Study the drawing (mm; zero at the part's minimum x, y, z) and answer. Give positions to 0.01 mm unless a question says otherwise; leave off trailing zeros. Write each loop counter-clockwise with the first axis right and the second up, starting at its lowest first coordinate (ties: lowest second). Pieces come first, ordered by that corner, then holes. Notation, with made-up numbers: (-2, 49) -> (54, 49) arc R27 cw to (54, 76) -> close; hole circle Ø4 at (37.5, 30.25). An arc over 180 degrees is marked (long way). One line per question, with ' | ' between items.
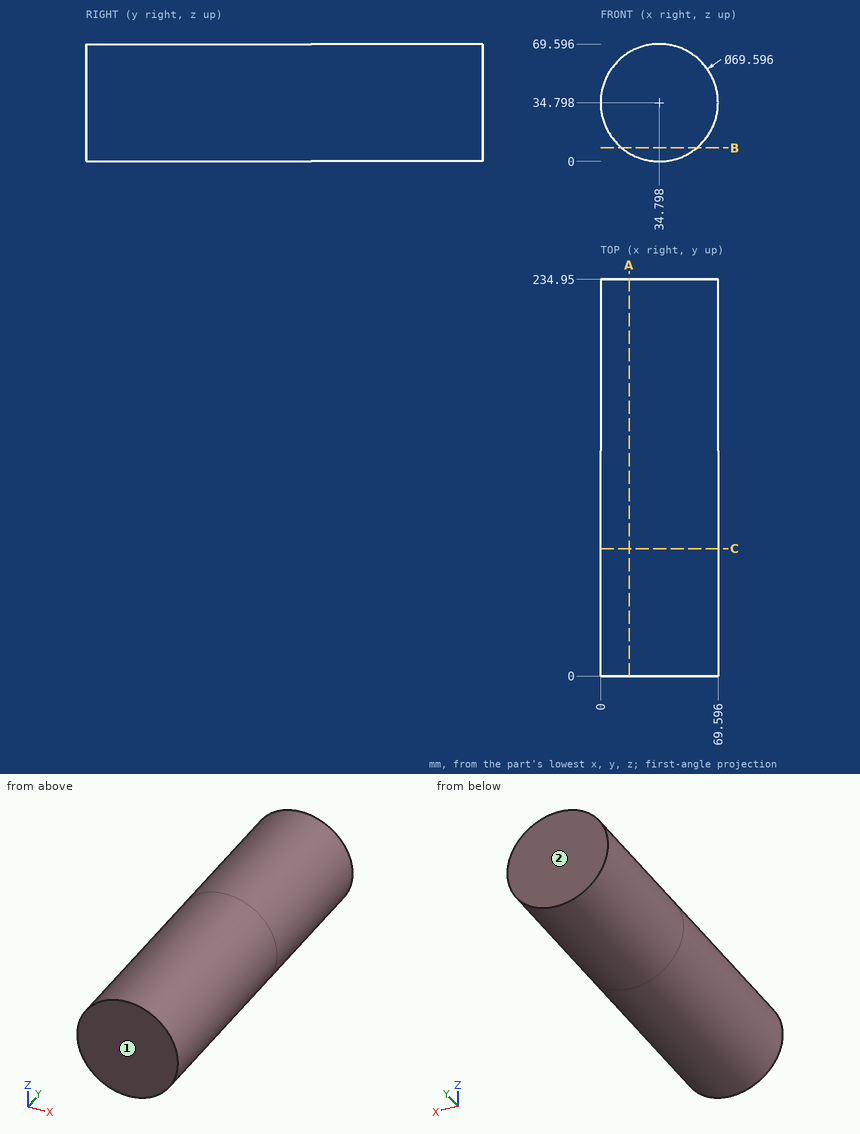
Item 1: Flat-ended cylindrical pins translate along their axes: pin 1 (1 mm diameter, centred on x = 17, y = 194.5, fed in from -Z); pin 2 (10 mm diameter, centred on x = 13, y = 118.5, fed in from +Z); pin 3 (6 mm diameter, centred on x = 24, y = 46, fed in from -Z) (3 decimals). Find the tip coordinate at first contact, or state that the pin passes through.
Answers below:
pin 1: z = 4.6 | pin 2: z = 65.27 | pin 3: z = 0.885
Item 2: Determine the mould class of the marked faces 1 and 2 for opening direction Y: pulls with the +Y half, pulls with the -Y half, needs draft (parallel to the pull), parting line crosses it, or undercut.
Answers below:
face 1: pulls with the -Y half | face 2: pulls with the +Y half
Item 3: Find section B-B (z = 8). Write down the section's boundary in (x, y).
Answers below:
outline: (12.6, 0) -> (57, 0) -> (57, 234.95) -> (12.6, 234.95) -> close
Item 4: Find section C-C (y = 75.5). Write down the section's boundary in (x, z), then the cut area to 3 significant figures.
Answers below:
outline: circle Ø69.6 at (34.8, 34.8) | area: 3,800 mm²
Item 5: Consider line 1 (Z direction, x = 35, y = 45); line 2 (X direction, y = 14, z = 34); line 3 (Z direction, x = 61, y = 206). Determine where each line is inside the solid, lowest interval first. Write a range as [from, to].
Answers below:
line 1: [0, 69.6] | line 2: [0.01, 69.59] | line 3: [11.9, 57.7]
Item 6: Find section A-A (x = 17). Write down the section's boundary in (y, z).
Answers below:
outline: (0, 4.9) -> (234.95, 4.9) -> (234.95, 64.7) -> (0, 64.7) -> close
